from build123d import *

# Parameters (mm, degrees)
SKETCH2_W                        = 30.56
SKETCH2_H                        = 22
BOSS_EXTRUDE1_DEPTH              = 27
SKETCH4_W                        = 28.75
SKETCH4_H                        = 12.5
CUT_EXTRUDE1_DEPTH               = 17
SKETCH5_W                        = 4
SKETCH5_H                        = 12.5
SKETCH5_H_2                      = 5
CUT_EXTRUDE2_DEPTH               = 39.032596546
SKETCH9_W                        = 27.5
SKETCH9_H                        = 18.5
BOSS_EXTRUDE2_DEPTH              = 30
FILLET1_R                        = 35
BOSS_EXTRUDE3_DEPTH              = 6
SKETCH10_6_W                     = 25.5
SKETCH10_6_H                     = 22.5
CUT_EXTRUDE3_DEPTH               = 51.80935839
SKETCH13_W                       = 22.5
SKETCH13_H                       = 2
BOSS_EXTRUDE4_DEPTH              = 25.5
SKETCH14_R                       = 3.5
CUT_EXTRUDE4_DEPTH               = 53.398386426
SKETCH20_W                       = 4
SKETCH20_H                       = 8.5
BOSS_EXTRUDE13_DEPTH             = 4
BOSS_EXTRUDE13_DIRECTION_2_REACH = 45.035
CUT_EXTRUDE5_START               = -4
SKETCH15_R                       = 1.125
CUT_EXTRUDE5_DEPTH               = 12
SKETCH21_W                       = 22
SKETCH21_H                       = 6.5
BOSS_EXTRUDE14_DEPTH             = 5
SKETCH22_W                       = 27.5
SKETCH22_H                       = 30
BOSS_EXTRUDE15_DEPTH             = 8


with BuildPart() as part:
    # Sketch2 → Boss-Extrude1 (new body)
    with BuildSketch(Plane(origin=(0, 0, 0), x_dir=(1, 0, 0), z_dir=(0, 1, 0))):
        Rectangle(SKETCH2_W, SKETCH2_H)
    extrude(amount=BOSS_EXTRUDE1_DEPTH)

    # Sketch4 → Cut-Extrude1 (cut)
    with BuildSketch(Plane.XY.offset(11)):
        with Locations((0.905, 8.25)):
            Rectangle(SKETCH4_W, SKETCH4_H)
    extrude(amount=-CUT_EXTRUDE1_DEPTH, mode=Mode.SUBTRACT)

    # Sketch5 → Cut-Extrude2 (cut, through all)
    with BuildSketch(Plane(origin=(0, 0, -11), x_dir=(-1, 0, 0), z_dir=(0, 0, -1))):
        with Locations((-2.03, 8.25)):
            Rectangle(SKETCH5_W, SKETCH5_H)
        with Locations((7.47, 7.5)):
            Rectangle(SKETCH5_W, SKETCH5_H_2)
    extrude(amount=-CUT_EXTRUDE2_DEPTH, mode=Mode.SUBTRACT)

    # Sketch9 → Boss-Extrude2 (add)
    with BuildSketch(Plane.ZY.offset(15.28)):
        with Locations((0, 17.75)):
            Rectangle(SKETCH9_W, SKETCH9_H)
    extrude(amount=BOSS_EXTRUDE2_DEPTH)

    # Fillet1
    # the kernel refuses this fillet: 35 mm, written as the material it takes off along each edge
    with BuildSketch(Plane(origin=(-45.28, 27, -90.91662167), x_dir=(1, 0, 0), z_dir=(0, 0, 1))) as fillet1_piece_1:
        with BuildLine():
            CenterArc((30.866648668, -35), FILLET1_R, 90, 61.872931781)
            Line((0, -18.5), (-0.617332973, -18.17))
            ThreePointArc((-0.617332973, -18.17), (-0.7, -9.25), (-0.7, 0))
            Line((-0.7, 0), (0, 0.7))
            Line((0, 0.7), (30.866648668, 0.7))
            Line((30.866648668, 0.7), (30.866648668, 0))
        make_face()
    extrude(amount=181.833243341, mode=Mode.SUBTRACT)

    # Sketch10 → Boss-Extrude3 (add)
    with BuildSketch(Plane.XZ.offset(-8.5)):
        Polygon((-45.28, 13.75), (-45.28, 11.25), (-19.78, 11.25), (-19.78, -11.25), (-45.28, -11.25), (-45.28, -13.75), (-17.78, -13.75), (-17.78, 13.75), align=None)
    extrude(amount=BOSS_EXTRUDE3_DEPTH)

    # Sketch10<6> → Cut-Extrude3 (cut, through all)
    with BuildSketch(Plane.XZ.offset(-8.5)):
        with Locations((-32.53, 0)):
            Rectangle(SKETCH10_6_W, SKETCH10_6_H)
    extrude(amount=-CUT_EXTRUDE3_DEPTH, mode=Mode.SUBTRACT)

    # Sketch13 → Boss-Extrude4 (add)
    with BuildSketch(Plane.ZY.offset(19.78)):
        with Locations((0, 3.5)):
            Rectangle(SKETCH13_W, SKETCH13_H)
    extrude(amount=BOSS_EXTRUDE4_DEPTH)

    # Sketch14 → Cut-Extrude4 (cut, through all)
    with BuildSketch(Plane(origin=(0, 4.5, 0), x_dir=(1, 0, 0), z_dir=(0, 1, 0))):
        with Locations(Location((-32.53, 0, 0), (0, 0, 270))):
            Circle(SKETCH14_R)
    extrude(amount=-CUT_EXTRUDE4_DEPTH, mode=Mode.SUBTRACT)

    # Sketch20 → Boss-Extrude13 (add)
    with BuildSketch(Plane.ZY.offset(15.28)):
        with Locations((11.75, 4.25)):
            Rectangle(SKETCH20_W, SKETCH20_H)
        with Locations((-11.75, 4.25)):
            Rectangle(SKETCH20_W, SKETCH20_H)
    extrude(amount=BOSS_EXTRUDE13_DEPTH)

    # Boss-Extrude13 direction 2: up to this face of the body (flat: up to its plane)
    boss_extrude13_direction_2_end = Plane(part.part.faces().sort_by_distance((-13.47, 8.25, 2.5))[0])
    # Sketch20 → Boss-Extrude13 direction 2 (add, up to the picked face)
    with BuildSketch(Plane.ZY.offset(15.28), mode=Mode.PRIVATE) as boss_extrude13_direction_2_sk1:
        with Locations((11.75, 4.25)):
            Rectangle(SKETCH20_W, SKETCH20_H)
    boss_extrude13_direction_2_tool1 = split(extrude(boss_extrude13_direction_2_sk1.sketch, amount=-BOSS_EXTRUDE13_DIRECTION_2_REACH, mode=Mode.PRIVATE), bisect_by=boss_extrude13_direction_2_end, keep=Keep.BOTH, mode=Mode.PRIVATE)
    # Sketch20 → Boss-Extrude13 direction 2 (add, up to the picked face)
    with BuildSketch(Plane.ZY.offset(15.28), mode=Mode.PRIVATE) as boss_extrude13_direction_2_sk2:
        with Locations((-11.75, 4.25)):
            Rectangle(SKETCH20_W, SKETCH20_H)
    boss_extrude13_direction_2_tool2 = split(extrude(boss_extrude13_direction_2_sk2.sketch, amount=-BOSS_EXTRUDE13_DIRECTION_2_REACH, mode=Mode.PRIVATE), bisect_by=boss_extrude13_direction_2_end, keep=Keep.BOTH, mode=Mode.PRIVATE)
    add(boss_extrude13_direction_2_tool1.solids().sort_by(Axis((-15.28, 4.25, 11.75), (1, 0, 0)))[0])
    add(boss_extrude13_direction_2_tool2.solids().sort_by(Axis((-15.28, 4.25, -11.75), (1, 0, 0)))[0])

    # Sketch15 → Cut-Extrude5 (cut)
    with BuildSketch(Plane(origin=(-17.78, 0, 0), x_dir=(0, 0, -1), z_dir=(1, 0, 0)).offset(CUT_EXTRUDE5_START)):
        with Locations(Location((-11.5, 2, 0), (0, 0, 153.612200039))):
            Circle(SKETCH15_R)
    cut_extrude5 = extrude(amount=CUT_EXTRUDE5_DEPTH, mode=Mode.SUBTRACT)

    # Mirror3: Cut-Extrude5 across plane
    add(cut_extrude5.mirror(Plane.XY), mode=Mode.SUBTRACT)

    # Sketch21 → Boss-Extrude14 (add)
    with BuildSketch(Plane(origin=(15.28, 0, 0), x_dir=(0, 0, -1), z_dir=(1, 0, 0))):
        with Locations((0, 23.75)):
            Rectangle(SKETCH21_W, SKETCH21_H)
    extrude(amount=BOSS_EXTRUDE14_DEPTH)

    # Sketch22 → Boss-Extrude15 (add)
    with BuildSketch(Plane(origin=(20.28, 0, 0), x_dir=(0, 0, -1), z_dir=(1, 0, 0))):
        with Locations((0, 35.5)):
            Rectangle(SKETCH22_W, SKETCH22_H)
    extrude(amount=-BOSS_EXTRUDE15_DEPTH)


solid = part.part
CAD build for the part. Positions are in the model's coordinates, mm. A direction names the side the tool comes from. Coordinates: 2 decimals unless noted, no trailing zeros. Write each loop counter-clockwise with the first axis right and the second up, starting at its lowest first coordinate (ties: lowest second). Pieces come first, ordered by that corner, then holes. Notation, with made-up numbers: M 10.25,14.25 L 52.25,14.25 A16 ccw 52.25,25.25 Z; hole C -17,1 d2. An arc over 180 degrees is marked long. Return JSON: item names as keys, results as strings.
Item 1: Drop flat-ended pins along their axis: pin 1 Ø21.5 at (x, y) = (-4.5, 19) entering from -Z; pin 2 Ø8 at (y, z) = (20, 0) entering from -X; pin 3 Ø3 at (x, z) = (-8.5, -7.5) entering from +Y; pin 4 Ø3 at (y, z) = (2, 11.5) entering from -X. Give the stop position or say it passes through.
Findings below:
{"pin 1": "stops at z = -11", "pin 2": "stops at x = -19.78", "pin 3": "stops at y = 27", "pin 4": "stops at x = -45.28"}
Item 2: Slice it at B-B, the plane x = -2.5. Write the cut outline in (y, z).
Findings below:
{"outline": "M 0,-11 L 27,-11 L 27,11 L 14.5,11 L 14.5,-6 L 2,-6 L 2,11 L 0,11 Z"}
Item 3: Two-plate mould, pull along Y, no slides. Class faces 5 (the flat face through (-30, 13, 11.25)), 6 (the flat face through (1, 14.5, 3)), 7 (the flat face through (-14, 8.5, -12)): +Y half, -Y half, draft (parallel to the pull), parting line (faces both ways), or undercut.
Findings below:
{"face 5": "draft", "face 6": "undercut", "face 7": "+Y half"}
Item 4: Which spindle directions (+Z, -Z, +X, -X, +Y, -Y) get a long thin tool onto all of the face, cutting with end or side? Do faces 1 (the flat face through (-19.78, 16, 0)), 2 (the flat face through (-7, 5, -9)), 3 (the flat face through (-5, 8, -6)), 4 (the flat face through (15.28, 15, -2)). Say none if no direction does.
Findings below:
{"face 1": "-X, +Y", "face 2": "+Z, -Z", "face 3": "+Z, +X", "face 4": "+Z, -Z, +X, -Y"}
Item 5: Slice it at C-C, the plane y = 11.5. Write the cut outline in (x, z), and give its area (3 significant figures).
Findings below:
{"outline": "M -43.48,-13.75 L -15.28,-13.75 L -15.28,-11 L 0.03,-11 L 0.03,-6 L -13.47,-6 L -13.47,11 L -15.28,11 L -15.28,13.75 L -43.48,13.75 L -43.48,11.25 L -19.78,11.25 L -19.78,-11.25 L -43.48,-11.25 Z; M 4.03,-11 L 15.28,-11 L 15.28,-6 L 4.03,-6 Z", "area": "406 mm2"}
Item 6: Slice it at D-D, the plane z = 7. Write the cut outline in (x, y), and give its area (3 significant figures).
Findings below:
{"outline": "M -45.28,2.5 L -17.78,2.5 L -17.78,8.5 L -15.28,8.5 L -15.28,0 L 15.28,0 L 15.28,2 L -13.47,2 L -13.47,14.5 L 15.28,14.5 L 15.28,20.5 L 20.28,20.5 L 20.28,50.5 L 12.28,50.5 L 12.28,27 L -14.41,27 A35 ccw -19.78,26.59 L -19.78,4.5 L -45.28,4.5 Z", "area": "832 mm2"}
Item 7: Slice it at A-A, the plane z = -2. Write the cut outline in (x, y), and give its area (3 significant figures).
Findings below:
{"outline": "M -45.28,2.5 L -35.4,2.5 L -35.4,4.5 L -45.28,4.5 Z; M -29.66,2.5 L -17.78,2.5 L -17.78,8.5 L -15.28,8.5 L -15.28,0 L 15.28,0 L 15.28,2 L -13.47,2 L -13.47,14.5 L 15.28,14.5 L 15.28,20.5 L 20.28,20.5 L 20.28,50.5 L 12.28,50.5 L 12.28,27 L -14.41,27 A35 ccw -19.78,26.59 L -19.78,4.5 L -29.66,4.5 Z", "area": "820 mm2"}
Item 8: Probe line 1 (X direction, y = 3.85, z = 0); line 2 (Y direction, x = -6.5, z = -6.25); line 3 (Y direction, x = -3, z = -5.5). List the from-to ranges inside material, lowest first. Write a range as from..to.
Findings below:
{"line 1": "x = -45.28..-36.03, -29.03..-17.78, -15.28..-13.47", "line 2": "y = 0..5, 10..27", "line 3": "y = 0..2, 14.5..27"}
